```python
from build123d import *

# Parameters (mm, degrees)
BOSS_EXTRUDE1_DEPTH = 12.7
HOLE3_D             = 3.175
HOLE3_DEPTH         = 31.75
HOLE3_CSINK_D       = 10.16
HOLE3_CSINK_ANGLE   = 82
HOLE3_TIP           = 0.953866233
HOLE6_D             = 3.175
HOLE6_DEPTH         = 38.1
HOLE6_CSINK_D       = 10.16
HOLE6_CSINK_ANGLE   = 82
HOLE6_TIP           = 0.953866233
HOLE7_D             = 3.175
HOLE7_DEPTH         = 31.75
HOLE7_CSINK_D       = 10.16
HOLE7_CSINK_ANGLE   = 82
HOLE7_TIP           = 0.953866233
HOLE8_D             = 3.175
HOLE8_DEPTH         = 31.75
HOLE8_CSINK_D       = 10.16
HOLE8_CSINK_ANGLE   = 82
HOLE8_TIP           = 0.953866233


with BuildPart() as part:
    # Sketch1 → Boss-Extrude1 (new body)
    with BuildSketch(Plane.XY):
        Polygon((-88.190159952, 0), (-222.052967181, 0), (-222.052967181, -248.25), (-64.977416983, -197.966048293), align=None)
    extrude(amount=-BOSS_EXTRUDE1_DEPTH)

    # Hole3
    with Locations(Plane(origin=(-234.752967181, 1090.512770337, -135.816741379), x_dir=(0, 0, -1), z_dir=(-1, 0, 0))):
        with Locations((-129.466741379, 1300.662770337), (-129.466741379, 1128.612770337), (129.198788767, 1128.612770337), (129.198788767, 1300.662770337)):
            CounterSinkHole(HOLE3_D / 2, HOLE3_CSINK_D / 2, depth=HOLE3_DEPTH, counter_sink_angle=HOLE3_CSINK_ANGLE)
            with Locations((0, 0, -(HOLE3_DEPTH + HOLE3_TIP / 2))):  # 118° drill point
                Cone(0, HOLE3_D / 2, HOLE3_TIP, mode=Mode.SUBTRACT)

    # Hole6
    with Locations(Plane(origin=(181.039434513, 1090.512770337, 0), x_dir=(-0.927183855, -0.374606593, 0), z_dir=(0, 0, 1))):
        with Locations((707.166557203, 1065.270372796), (674.127983646, 944.603090451)):
            CounterSinkHole(HOLE6_D / 2, HOLE6_CSINK_D / 2, depth=HOLE6_DEPTH, counter_sink_angle=HOLE6_CSINK_ANGLE)
            with Locations((0, 0, -(HOLE6_DEPTH + HOLE6_TIP / 2))):  # 118° drill point
                Cone(0, HOLE6_D / 2, HOLE6_TIP, mode=Mode.SUBTRACT)

    # Hole7
    with Locations(Plane(origin=(181.039434513, 12.7, -135.816741379), x_dir=(0, 0, -1), z_dir=(0, 1, 0))):
        with Locations((129.198788767, 384.042401694), (-129.466741379, 384.042401694), (-129.466741379, 304.786761906), (-110.416741379, 409.442401694), (-0.133976306, 409.442401694), (110.148788767, 409.442401694), (129.198788767, 304.786761906)):
            CounterSinkHole(HOLE7_D / 2, HOLE7_CSINK_D / 2, depth=HOLE7_DEPTH, counter_sink_angle=HOLE7_CSINK_ANGLE)
            with Locations((0, 0, -(HOLE7_DEPTH + HOLE7_TIP / 2))):  # 118° drill point
                Cone(0, HOLE7_D / 2, HOLE7_TIP, mode=Mode.SUBTRACT)

    # Hole8
    with Locations(Plane(origin=(536.177050645, -18.855816567, -135.816741379), x_dir=(0, 0, 1), z_dir=(0.304884492, -0.952389336, 0))):
        with Locations((-129.257383629, 766.263727577), (129.466741379, 668.242950575), (129.466741379, 766.064256541), (-129.408220012, 668.442537903)):
            CounterSinkHole(HOLE8_D / 2, HOLE8_CSINK_D / 2, depth=HOLE8_DEPTH, counter_sink_angle=HOLE8_CSINK_ANGLE)
            with Locations((0, 0, -(HOLE8_DEPTH + HOLE8_TIP / 2))):  # 118° drill point
                Cone(0, HOLE8_D / 2, HOLE8_TIP, mode=Mode.SUBTRACT)


solid = part.part
```
Source: CAD feature listing. Evaluate the final solid. Frame: model axes, mm. Give positions to 0.01 mm unless a question says otherwise; leave off trailing zeros. Write each loop counter-clockwise with the first axis right and the second up, starting at its lowest first coordinate (ties: lowest second). Pieces come first, ordered by that corner, then holes.
1. Section query A-A (y = -216). Return the cut outline in (x, z).
2. Section query B-B (x = -116). Return the cut outline in (y, z), then the cut area to 3 significant figures.
3. Pull-direction query (X, two-part tool) for faces 1 (the face through (-76.42, -100.37, -6.26)), 2 (the face through (-145, -122, -12.7)), 3 (the face through (-108.566, -201.779, -6.143)); classes: +X half, -X half, draft (parallel to the pull), parting line (faces both ways), or undercut.
4. Material intervals for line 1 along Y through (x, z) = (-215.25, -6.35); line 2 along Y through (x, z) = (-214, -6.35); line 3 along Z through (x, y) = (-214.5, -38.1), sorted ascending.
5. First-contact query: pin 1 (6 mm diameter, centred on x = -164, y = -68.5, fed in from +Z); pin 2 (2.5 mm diameter, centred on x = -203, z = -6.35, fed in from +Y); pin 3 (5 mm diameter, centred on y = -38.1, z = -6.35, fed in from +X); pin 4 (3.5 mm diameter, centred on x = -123.75, z = -6.35, fed in from -Y). Flat tips, straight axial feed; report the tip coordinate or a pass-through.
Output values:
1. outline: (-222.05, -12.7) - (-121.31, -12.7) - (-121.31, 0) - (-222.05, 0) - close
2. outline: (-214.3, -12.7) - (0, -12.7) - (0, 0) - (-214.3, 0) - close
2. area: 2,720 mm2
3. face 1: +X half
3. face 2: draft
3. face 3: undercut
4. line 1: y = -246.07 to -211.74, -208.56 to -39.69, -36.51 to 0
4. line 2: y = -245.67 to -211.74, -208.56 to -39.69, -36.51 to 0
4. line 3: z = -12.7 to -7.94, -4.76 to 0
5. pin 1: stops at z = 0
5. pin 2: stops at y = -19.25
5. pin 3: stops at x = -83.43
5. pin 4: stops at y = -217.34
